from build123d import *

# Parameters (mm, degrees)
SALIENTE_EXTRUIR2_DEPTH = 17
CROQUIS4_R              = 7.575
CORTAR_EXTRUIR7_DEPTH   = 18
CROQUIS12_R             = 5.075
CORTAR_EXTRUIR12_DEPTH  = 18
CROQUIS17_R             = 1.75
CORTAR_EXTRUIR15_DEPTH  = 18
CORTAR_EXTRUIR9_DEPTH   = 14
CORTAR_EXTRUIR10_DEPTH  = 15
CROQUIS10_R             = 2.675
CORTAR_EXTRUIR11_DEPTH  = 8.6
SALIENTE_EXTRUIR3_DEPTH = 15
SALIENTE_EXTRUIR4_DEPTH = 15
CROQUIS16_R             = 2.675
CORTAR_EXTRUIR14_DEPTH  = 8.6
CROQUIS18_W             = 23
CROQUIS18_H             = 25
CORTAR_EXTRUIR16_DEPTH  = 7
CORTAR_EXTRUIR17_DEPTH  = 2.5
REDONDEO2_R             = 1
REDONDEO4_R             = 2


with BuildPart() as part:
    # Croquis1 → Saliente-Extruir2 (new body)
    with BuildSketch(Plane(origin=(0, 0, 0), x_dir=(1, 0, 0), z_dir=(0, 1, 0))):
        Polygon((23, -63.5), (23, -23), (43, -23), (43, 0), (0, 0), (0, -63.5), align=None)
    extrude(amount=-SALIENTE_EXTRUIR2_DEPTH)

    # Croquis4 → Cortar-Extruir7 (cut, through all)
    with BuildSketch(Plane(origin=(0, 0, 0), x_dir=(-1, 0, 0), z_dir=(0, -1, 0))):
        with Locations((-11.5, -10)):
            Circle(CROQUIS4_R)
    extrude(amount=CORTAR_EXTRUIR7_DEPTH, mode=Mode.SUBTRACT)

    # Croquis12 → Cortar-Extruir12 (cut, through all)
    with BuildSketch(Plane(origin=(0, 0, 0), x_dir=(1, 0, 0), z_dir=(0, 1, 0))):
        with Locations((11.5, -32)):
            Circle(CROQUIS12_R)
    extrude(amount=-CORTAR_EXTRUIR12_DEPTH, mode=Mode.SUBTRACT)

    # Croquis17 → Cortar-Extruir15 (cut, through all)
    with BuildSketch(Plane(origin=(0, 0, 0), x_dir=(1, 0, 0), z_dir=(0, 1, 0))):
        with Locations((11.5, -24)):
            Circle(CROQUIS17_R)
        with Locations((11.5, -40)):
            Circle(CROQUIS17_R)
        with Locations((3.5, -32)):
            Circle(CROQUIS17_R)
        with Locations((19.5, -32)):
            Circle(CROQUIS17_R)
    extrude(amount=-CORTAR_EXTRUIR15_DEPTH, mode=Mode.SUBTRACT)

    # Croquis8 → Cortar-Extruir9 (cut)
    with BuildSketch(Plane(origin=(43, 0, 0), x_dir=(0, 0, -1), z_dir=(1, 0, 0))):
        Polygon((0, -17), (0, 0), (-16.5, 0), (-16.5, -1.4), (-1.4, -1.4), (-1.4, -17), align=None)
    extrude(amount=-CORTAR_EXTRUIR9_DEPTH, mode=Mode.SUBTRACT)

    # Croquis9 → Cortar-Extruir10 (cut)
    with BuildSketch(Plane(origin=(0, 0, 63.5), x_dir=(-1, 0, 0), z_dir=(0, 0, -1))):
        Polygon((0, -17), (-1.4, -17), (-1.4, -1.4), (-16.5, -1.4), (-16.5, 0), (0, 0), align=None)
    extrude(amount=CORTAR_EXTRUIR10_DEPTH, mode=Mode.SUBTRACT)

    # Croquis10 → Cortar-Extruir11 (cut)
    with BuildSketch(Plane(origin=(0, -1.4, 0), x_dir=(1, 0, 0), z_dir=(0, 1, 0))):
        with Locations((36.75, -8.95)):
            Circle(CROQUIS10_R)
        with Locations((8.95, -56)):
            Circle(CROQUIS10_R)
    extrude(amount=-CORTAR_EXTRUIR11_DEPTH, mode=Mode.SUBTRACT)

    # Croquis14 → Saliente-Extruir3 (add)
    with BuildSketch(Plane.XY.offset(63.5)):
        Polygon((23, 0), (16.5, 0), (16.5, -1.4), (1.4, -1.4), (1.4, -17), (23, -17), align=None)
    extrude(amount=SALIENTE_EXTRUIR3_DEPTH)

    # Croquis15 → Saliente-Extruir4 (add)
    with BuildSketch(Plane(origin=(43, 0, 0), x_dir=(0, 0, -1), z_dir=(1, 0, 0))):
        Polygon((-1.4, -17), (-1.4, -1.4), (-16.5, -1.4), (-16.5, 0), (-23, 0), (-23, -17), align=None)
    extrude(amount=SALIENTE_EXTRUIR4_DEPTH)

    # Croquis16 → Cortar-Extruir14 (cut)
    with BuildSketch(Plane(origin=(0, -1.4, 0), x_dir=(1, 0, 0), z_dir=(0, 1, 0))):
        with Locations((8.95, -71)):
            Circle(CROQUIS16_R)
        with Locations((51.75, -8.95)):
            Circle(CROQUIS16_R)
    extrude(amount=-CORTAR_EXTRUIR14_DEPTH, mode=Mode.SUBTRACT)

    # Croquis18 → Cortar-Extruir16 (cut)
    with BuildSketch(Plane.XZ.offset(17)):
        with Locations((11.5, 32)):
            Rectangle(CROQUIS18_W, CROQUIS18_H)
    extrude(amount=-CORTAR_EXTRUIR16_DEPTH, mode=Mode.SUBTRACT)

    # Croquis19 → Cortar-Extruir17 (cut)
    with BuildSketch(Plane.XZ.offset(10)):
        Polygon((14.675426481, 40), (13.08771324, 42.75), (9.91228676, 42.75), (8.324573519, 40), (9.91228676, 37.25), (13.08771324, 37.25), align=None)
        Polygon((22.25, 30.41228676), (22.25, 33.58771324), (19.5, 35.175426481), (16.75, 33.58771324), (16.75, 30.41228676), (19.5, 28.824573519), align=None)
        Polygon((14.675426481, 24), (13.08771324, 26.75), (9.91228676, 26.75), (8.324573519, 24), (9.91228676, 21.25), (13.08771324, 21.25), align=None)
        Polygon((0.75, 33.58771324), (0.75, 30.41228676), (3.5, 28.824573519), (6.25, 30.41228676), (6.25, 33.58771324), (3.5, 35.175426481), align=None)
    extrude(amount=-CORTAR_EXTRUIR17_DEPTH, mode=Mode.SUBTRACT)

    # Redondeo2
    redondeo2_edges = [part.edges().sort_by_distance(p)[0] for p in [
        (23, -13.5, 23),
        (23, -13.5, 44.5),
        (0, -13.5, 44.5),
        (23, -13.5, 19.5),
        (0, -13.5, 19.5),
    ]]
    fillet(redondeo2_edges, radius=REDONDEO2_R)

    # Redondeo4
    redondeo4_edges = [part.edges().sort_by_distance(p)[0] for p in [
        (43.5, -1.4, 1.4),
        (1.4, -1.4, 63.5),
    ]]
    fillet(redondeo4_edges, radius=REDONDEO4_R)


solid = part.part
CAD build for the part. Positions are in the model's coordinates, mm. A direction names the side the tool comes from. Coordinates: 2 decimals unless noted, no trailing zeros. Loops run counter-clockwise (first coordinate to the right, second up) from the corner with the lowest first, then second, coordinate; pieces in that order, holes last. Notation, with made-up numbers: (87, 32) - (102, 32) arc R12 ccw to (102, 41) - close; hole circle Ø5 at (-37.75, 57). An arc over 180 degrees is marked (long way). Use one line per item in the form item = value. Start each with the question number.
1) Drill centre lines: L1, parallel to Z at x = 11, y = -15.5; L2, parallel to X at y = -10.75, z = 10 (3 decimals); L3, parallel to Z at x = 3.5, y = -6. Where is each one in solid material? Low to high. Write a range as from..to.
2) Band-saw the part on A-A (y = -12.5). Give the cut face in (x, z) (3 decimals), and give its area (3 significant figures).
3) Band-saw the part on B-B (x = 45). Give the cut face in (y, z), and give its area (3 significant figures).
4) Flat gauge pins, fed straight in: pin 1 (3 mm diameter, centred on x = 3.5, z = 32, fed in from -Y); pin 2 (1.2 mm diameter, centred on y = -9, z = 31.5, fed in from +X); pin 3 (7 mm diameter, centred on x = 13, z = 38, fed in from -Y); pin 4 (6 mm diameter, centred on x = 36.5, z = 9, fed in from +Y). Where does each tip first touch, or does it go through?
5) Band-saw the part on D-D (y = -4.75). State how many separate pieces and enclosed holes the cut face has, and give its area (3 significant figures).
6) Tool access for faces 4 (the face through (37, -10, 9)), 5 (the face through (1.4, -10, 63)), 6 (the face through (11, -14, 44.5)), 7 (the face through (23, -14, 21)), 8 (the face through (13.89, -8.77, 41.36)): list every direction of +Z, -Z, +X, -X, +Y, -Y with a clear straight run to the whole face (end or side of a thin tool).
7) Two-plate mould, pull along Z, no slides. Class faces 1 (the face through (12.9, -7.5, 41.3)), 2 (the face through (35, -17, 12)), 3 (the face through (43.7, -1.97, 2)): +Z half, -Z half, draft (parallel to the pull), parting line (faces both ways), or undercut.
8) Band-saw the part on C-C (z = 56). Give the cut face in (x, y) (3 decimals), and give its area (3 significant figures).
Check values:
q1.L1 = 0..2.44, 17.56..19.5, 44.5..78.5
q1.L2 = 0..3.925, 19.075..58
q1.L3 = 0..30.25, 33.75..78.5
q2.outline = (0, 0) - (29, 0) - (29, 1.4) - (58, 1.4) - (58, 23) - (24, 23) arc R1 ccw to (23, 22) - (23, 20.5) arc R1 cw to (22, 19.5) - (1, 19.5) arc R1 ccw to (0, 18.5) - close; (0, 45.5) arc R1 ccw to (1, 44.5) - (22, 44.5) arc R1 ccw to (23, 45.5) - (23, 78.5) - (1.4, 78.5) - (1.4, 48.5) - (0, 48.5) - close; hole circle Ø15.15 at (11.5, 10)
q2.area = 1,770 mm2
q3.outline = (-17, 1.4) - (-3.4, 1.4) arc R2 ccw to (-1.4, 3.4) - (-1.4, 16.5) - (0, 16.5) - (0, 23) - (-17, 23) - close
q3.area = 345 mm2
q4.pin_1 = through
q4.pin_2 = 23
q4.pin_3 = -10
q4.pin_4 = -1.4
q5.separate_pieces = 1
q5.enclosed_holes = 10
q5.area = 2,140 mm2
q6.face_4 = +Y
q6.face_5 = +Z, -X, +Y, -Y
q6.face_6 = +X, -X, -Y
q6.face_7 = -X, -Y
q6.face_8 = -Y
q7.face_1 = undercut
q7.face_2 = draft
q7.face_3 = -Z half
q8.outline = (1.4, -17) - (23, -17) - (23, 0) - (16.5, 0) - (16.5, -1.4) - (11.625, -1.4) - (11.625, -10) - (6.275, -10) - (6.275, -1.4) - (3.4, -1.4) arc R2 ccw to (1.4, -3.4) - close
q8.area = 299 mm2
